Work out the finished part from the listing and answer in its coordinate system (mm). A direction names the side the tool comes from. Round coordinates to 2 decimals unless told otherwise and drop trailing zeros. Write each loop counter-clockwise with the first axis right and the second up, starting at its lowest first coordinate (ties: lowest second). Pieces come first, ordered by that corner, then holes. Notation, with made-up numbers: M 33.25,-17 L 88.25,-17 A21 ccw 88.25,11 Z; hole C 2.25,63.5 d6. An arc over 180 degrees is marked long. Answer in a Markdown table with one row per item.
```python
from build123d import *

# Parameters (mm, degrees)
F0_W     = 20
F0_H     = 20
F1_DEPTH = 14
F3_DEPTH = 25
F5_D     = 5.2
F6_R     = 1
F7_R     = 1


with BuildPart() as f1:
    # F0 (on Top) → F1 (new body)
    with BuildSketch(Plane.XY):
        with Locations((10, 10)):
            Rectangle(F0_W, F0_H)
    extrude(amount=F1_DEPTH)

    # F2 (on Front) → F3 (join)
    with BuildSketch(Plane.XZ):
        with BuildLine():
            ThreePointArc((-20, 7), (10, 2.4258640188), (40, 7))
            ThreePointArc((40, 7), (10, 11.5741359812), (-20, 7))
        make_face()
    extrude(amount=F3_DEPTH)

    # F5 (through all)
    with Locations(Plane.XY.offset(14)):
        with Locations((10, 10)):
            Hole(F5_D / 2)

    # F6
    f6_edges = [f1.edges().sort_by_distance(p)[0] for p in [
        (40, -12.5, 7),
    ]]
    fillet(f6_edges, radius=F6_R)

    # F7
    f7_edges = [f1.edges().sort_by_distance(p)[0] for p in [
        (-20, -12.5, 7),
    ]]
    fillet(f7_edges, radius=F7_R)


solid = f1.part
```
1. The part is cut by section D-D (x = 3). Determine the outline of the cut face in (y, z), plus the area to 3 significant figures.
Calculated:
| item | result |
|---|---|
| outline | M -25,2.67 L 0,2.67 L 0,0 L 20,0 L 20,14 L 0,14 L 0,11.33 L -25,11.33 Z |
| area | 497 mm² |
2. The part is cut by section A-A (x = 10). Determine the outline of the cut face in (y, z).
Calculated:
| item | result |
|---|---|
| outline | M -25,2.43 L 0,2.43 L 0,0 L 7.4,0 L 7.4,14 L 0,14 L 0,11.57 L -25,11.57 Z; M 12.6,0 L 20,0 L 20,14 L 12.6,14 Z |
3. Consider line 1 along Y through (x, z) = (10, 5); line 2 along Y through (x, z) = (-6, 6.5); line 3 along Z through (x, y) = (0, -17). Determine where each line is inside the solid, lowest interval first. Write a range as from..to.
Calculated:
| item | result |
|---|---|
| line 1 | y = -25..7.4, 12.6..20 |
| line 2 | y = -25..0 |
| line 3 | z = 2.92..11.08 |
4. The part is cut by section C-C (z = 4). Determine the outline of the cut face in (x, y).
Calculated:
| item | result |
|---|---|
| outline | M -7.73,-25 L 27.73,-25 L 27.73,0 L 20,0 L 20,20 L 0,20 L 0,0 L -7.73,0 Z; hole C 10,10 d5.2 |
5. Given pin 1 (5 mm diameter, centred on x = 21, y = -17.5, fed in from +Z); pin 2 (1 mm diameter, centred on y = -9, z = 6, fed in from +X); pin 3 (5 mm diameter, centred on x = -6, y = -10, fed in from +Z), each flat-ended and moving along its own axis, determine where each tip first touches the part or whether it passes through.
Calculated:
| item | result |
|---|---|
| pin 1 | stops at z = 11.21 |
| pin 2 | stops at x = 37.32 |
| pin 3 | stops at z = 10.66 |
6. A tool of negligible diameter and unlimited length cuts with its end or side. For faces 1 (the flat face through (12, 12, 14)), 2 (the cylindrical face through (9.621, -12.325, 2.427)), 3 (the flat face through (-7, 0, 7)), 4 (the flat face through (20, 10, 7)), from which of +Z, -Z, +X, -X, +Y, -Y can it reach the whole face along a straight path? Write none if from no direction.
Calculated:
| item | result |
|---|---|
| face 1 | +Z, +X, -X, +Y, -Y |
| face 2 | -Z, -Y |
| face 3 | +Z, -Z, -X, +Y |
| face 4 | +Z, -Z, +X, +Y |
7. The part is cut by section B-B (y = 10). Determine the outline of the cut face in (x, z).
Calculated:
| item | result |
|---|---|
| outline | M 0,0 L 7.4,0 L 7.4,14 L 0,14 Z; M 12.6,0 L 20,0 L 20,14 L 12.6,14 Z |
8. Determine the mould class of faces 5 (the flat face through (0, 10, 7)), 6 (the flat face through (10, 0, 13)), 7 (the cylindrical face through (8.8, 7.693, 6.902)), 8 (the cylindrical face through (10.379, -12.325, 11.573)) for opening direction X: released by +X, released by -X, zero draft, split by the parting line, or undercut.
Calculated:
| item | result |
|---|---|
| face 5 | released by -X |
| face 6 | zero draft |
| face 7 | undercut |
| face 8 | split by the parting line |
